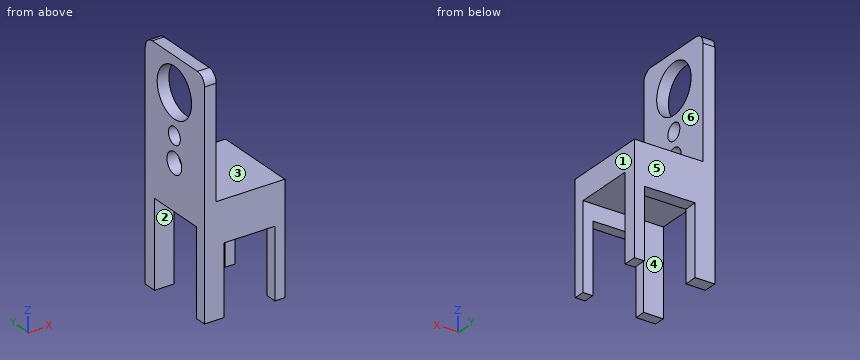
```python
from build123d import *

# Parameters (mm, degrees)
F0_R     = 6.6404165098
F0_R_2   = 5.3780790225
F0_R_3   = 15.463703615
F1_DEPTH = 3.683
F2_W     = 53.2784113497
F2_H     = 69.0371559083
F3_DEPTH = 42.926
F4_W     = 37.8411058336
F4_H     = 53.5067310557
F5_DEPTH = 50.293
F6_W     = 31.9212079048
F6_H     = 43.5216361657
F7_DEPTH = 53.2794113497


# Not quite as in the source:
# - a feature names something its author has since deleted; it is built from what else it names


with BuildPart() as f1:
    # F0 (on Right) → F1 (new body, symmetric)
    with BuildSketch(Plane.YZ):
        with BuildLine():
            Line((19.8416914791, 85.8998820186), (-20.7367198706, 85.8998820186))
            ThreePointArc((-20.7367198706, 85.8998820186), (-25.2268479311, 84.0400100791), (-27.0867198706, 79.5498820186))
            Line((-27.0867198706, 79.5498820186), (-27.0867198706, -58.5244297981))
            Line((-27.0867198706, -58.5244297981), (26.1916914791, -58.5244297981))
            Line((26.1916914791, -58.5244297981), (26.1916914791, 79.5498820186))
            ThreePointArc((26.1916914791, 79.5498820186), (24.3318195396, 84.0400100791), (19.8416914791, 85.8998820186))
        make_face()
        with Locations((0, 23.3183521777)):
            Circle(F0_R, mode=Mode.SUBTRACT)
        with Locations((0, 39.2750576138)):
            Circle(F0_R_2, mode=Mode.SUBTRACT)
        with Locations((0, 64.4399300218)):
            Circle(F0_R_3, mode=Mode.SUBTRACT)
    extrude(amount=F1_DEPTH, both=True)

    # F2 (on face) → F3 (join)
    with BuildSketch(Plane.YZ.offset(3.683)):
        with Locations((-0.4475141957, -24.005851844)):
            Rectangle(F2_W, F2_H)
    extrude(amount=F3_DEPTH)

    # F4 (on face) → F5 (cut, through all)
    with BuildSketch(Plane.YZ.offset(46.609)):
        with Locations((-1.2208549306, -31.7710642703)):
            Rectangle(F4_W, F4_H)
    extrude(amount=-F5_DEPTH, mode=Mode.SUBTRACT)

    # F6 (on face) → F7 (cut, through all)
    with BuildSketch(Plane(origin=(0, 26.1916914791, 0), x_dir=(-1, 0, 0), z_dir=(0, 1, 0))):
        with Locations((-24.5076268911, -36.7636117153)):
            Rectangle(F6_W, F6_H)
    extrude(amount=-F7_DEPTH, mode=Mode.SUBTRACT)


solid = f1.part
```
Check sheet for the modelled part. Datum: model origin and axes. Units: mm. Face numbers are marked on the shaded views. A direction names the side the tool comes from. Give positions to 0.01 mm unless a question says otherwise; leave off trailing zeros. Write each loop counter-clockwise with the first axis right and the second up, starting at its lowest first coordinate (ties: lowest second). Pieces come first, ordered by that corner, then holes. Notation, with made-up numbers: (3.5, 85) - (61.5, 85) arc R33 ccw to (61.5, 119) - close; hole circle Ø4 at (15, 14). An arc over 180 degrees is marked (long way). Answer as a JSON object with one key per item and string values. Group by question number.
1) Sectioned sample at D-D (x = 15.5). Record the cut outline in (y, z).
2) Sectioned sample at A-A (y = 0). Record the cut outline in (x, z).
3) Thickness scan on probe 1 along Z at (x, y) = (-1, 0); probe 2 along Y at (x, z) = (19, -8); probe 3 along Z at (x, y) = (3.5, -4). Record the ranges inside material, lowest first. Write a range as from..to.
4) Sectioned sample at B-B (z = 74). Record the cut outline in (x, y), then the cut area to 3 significant figures.
5) Depth check by flat-ended pin: P1, Ø1.5, axis at x = 32, y = -12, coming from the +Z side; P2, Ø19, axis at x = 16.5, y = 2, coming from the -Z side; P3, Ø9.5, axis at x = 17.5, y = 24, coming from the -Z side. Enter the tip coordinate at first touch or a pass-through.
6) Access from +Z, -Z, +X, -X, +Y, -Y to the whole of each face (thin tool, end or side, straight path). Record for the marked faces 1, 2 and 3.
7) Release check for a two-part mould opening along Y. For the marked faces 4, 5 and 6 record: pulls with the +Y half, pulls with the -Y half, needs draft (parallel to the pull), parting line crosses it, or undercut.
8) Sectioned sample at C-C (y = -11.5). Record the cut outline in (x, z), then the cut area to 3 significant figures.
Geometry results:
{
 "1": {"outline": "(-27.09, -15) - (-20.14, -15) - (-20.14, -5.02) - (17.7, -5.02) - (17.7, -15) - (26.19, -15) - (26.19, 10.51) - (-27.09, 10.51) - close"},
 "2": {"outline": "(-3.68, -5.02) - (46.61, -5.02) - (46.61, 10.51) - (3.68, 10.51) - (3.68, 16.68) - (-3.68, 16.68) - close; (-3.68, 29.96) - (3.68, 29.96) - (3.68, 33.9) - (-3.68, 33.9) - close; (-3.68, 44.65) - (3.68, 44.65) - (3.68, 48.98) - (-3.68, 48.98) - close; (-3.68, 79.9) - (3.68, 79.9) - (3.68, 85.9) - (-3.68, 85.9) - close"},
 "3": {"probe 1": "z = -5.02..16.68, 29.96..33.9, 44.65..48.98, 79.9..85.9", "probe 2": "y = -27.09..-20.14, 17.7..26.19", "probe 3": "z = -5.02..18.02, 28.62..35.68, 42.87..49.5, 79.38..85.9"},
 "4": {"outline": "(-3.68, -27.09) - (3.68, -27.09) - (3.68, -12.15) - (-3.68, -12.15) - close; (-3.68, 12.15) - (3.68, 12.15) - (3.68, 26.19) - (-3.68, 26.19) - close", "area": "213 mm^2"},
 "5": {"P1": "stops at z = 10.51", "P2": "stops at z = -5.02", "P3": "stops at z = -15"},
 "6": {"face 1": "+Z, -Z, +X, +Y, -Y", "face 2": "-Z, +X, -X", "face 3": "+Z, +X, +Y, -Y"},
 "7": {"face 4": "undercut", "face 5": "pulls with the +Y half", "face 6": "needs draft"},
 "8": {"outline": "(-3.68, -5.02) - (46.61, -5.02) - (46.61, 10.51) - (3.68, 10.51) - (3.68, 54.1) - (-3.68, 54.1) - close; (-3.68, 74.78) - (3.68, 74.78) - (3.68, 85.9) - (-3.68, 85.9) - close", "area": "1,180 mm^2"}
}
